Here's how the part is built. I have some questions about the finished solid (model axes, mm). Round coordinates to 2 decimals unless told otherwise and drop trailing zeros. Loops run counter-clockwise (first coordinate to the right, second up) from the corner with the lowest first, then second, coordinate; pieces in that order, holes last. Notation, with made-up numbers: M 23.25,-7 L 49.25,-7 A17 ccw 49.25,4 Z; hole C 32.5,88.5 d1. An arc over 180 degrees is marked long. Use a Markdown table: item, result.
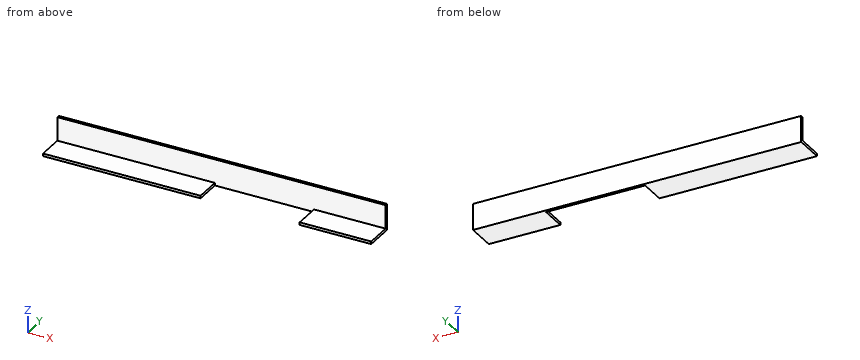
from build123d import *

# Parameters (mm, degrees)
F0_W     = 250
F0_H     = 2
F0_H_2   = 18
F1_DEPTH = 2
F2_DEPTH = 22
F3_W     = 75.5
F3_H     = 2
F4_DEPTH = 20


with BuildPart() as f1:
    # F0 (on Front) → F1 (new body)
    with BuildSketch(Plane.XZ):
        with Locations((125, 1)):
            Rectangle(F0_W, F0_H)
        with Locations((125, 11)):
            Rectangle(F0_W, F0_H_2)
    extrude(amount=F1_DEPTH)

    # F0 (on Front) → F2 (join)
    with BuildSketch(Plane.XZ):
        with Locations((125, 1)):
            Rectangle(F0_W, F0_H)
    extrude(amount=F2_DEPTH)

    # F3 (on face) → F4 (cut, through all)
    with BuildSketch(Plane.XZ.offset(22)):
        with Locations((157.75, 1)):
            Rectangle(F3_W, F3_H)
    extrude(amount=-F4_DEPTH, mode=Mode.SUBTRACT)


solid = f1.part
1. For pin 1 Ø1 at (x, z) = (79, 13) entering from -Y, with a flat end and sliding along its axis, tell me the tip position at first contact or that it passes through.
Answer sheet:
| item | result |
|---|---|
| pin 1 | y = -2 |
2. Imagine slicing it at D-D, the plane x = 176. Write out the boundary of the cut face in (y, z).
Answer sheet:
| item | result |
|---|---|
| outline | M -2,0 L 0,0 L 0,20 L -2,20 Z |
3. Imagine slicing it at B-B, the plane x = 231. Write out the boundary of the cut face in (y, z).
Answer sheet:
| item | result |
|---|---|
| outline | M -22,0 L 0,0 L 0,20 L -2,20 L -2,2 L -22,2 Z |
4. I need wall thicknesses on probe 1 along Z at (x, y) = (82.5, -16.25); probe 2 along Y at (x, z) = (27.5, 8.75). Which ranges of each line are inside material? Lowest first, please. Write a range as from..to.
Answer sheet:
| item | result |
|---|---|
| probe 1 | 0..2 |
| probe 2 | -2..0 |
5. Imagine slicing it at A-A, the plane y = -11.5. Write out the boundary of the cut face in (x, z), then the cut area to 3 significant figures.
Answer sheet:
| item | result |
|---|---|
| outline | M 0,0 L 120,0 L 120,2 L 0,2 Z; M 195.5,0 L 250,0 L 250,2 L 195.5,2 Z |
| area | 349 mm2 |
6. Imagine slicing it at C-C, the plane z = 10.25. Write out the boundary of the cut face in (x, y), then the cut area to 3 significant figures.
Answer sheet:
| item | result |
|---|---|
| outline | M 0,-2 L 250,-2 L 250,0 L 0,0 Z |
| area | 500 mm2 |
